Source: three-view drawing plus pictorial views. Frame: mm from the lowest corner of the part. A direction names the side the tool comes from. Round coordinates to 2 decimals unless told otherwise and drop trailing zeros. Loops run counter-clockwise (first coordinate to the right, second up) from the corner with the lowest first, then second, coordinate; pieces in that order, holes last. Notation, with made-up numbers: M 19.25,20.25 L 75.25,20.25 A19 ccw 75.25,56.25 Z; hole C 24.25,-16 d11. An arc over 180 degrees is marked long. Return JSON: item names as keys, results as strings. Group by question number.
1) Contact query for a flat-ended pin moving along its axis: P1, Ø1.5, axis at y = 45.5, z = 15.5, coming from the -X side. Output: stop coordinate, or through.
2) Material intervals for line 1 (X direction, y = 79, z = 18.5); line 2 (Y direction, x = 38.5, z = 9.25); line 3 (Y direction, x = 14.5, z = 3), sorted ascending. Write a range as from..to.
3) Section D-D (z = 2). Output: boundary loops of the cut face in (x, y).
4) Section B-B (z = 8.25). Output: boundary loops of the cut face in (x, y), plus the area to 3 significant figures.
5) Section C-C (y = 16.5). Output: boundary loops of the cut face in (x, z).
6) Access query for the marked faces 1 and 2. Directions: +Z, -Z, +X, -X, +Y, -Y. A direction counts if a zero-diameter tool reaches every point of the face in a straight line with its end or side. Return the directions, or none.
7) Section A-A (y = 140.5). Output: boundary loops of the cut face in (x, z).
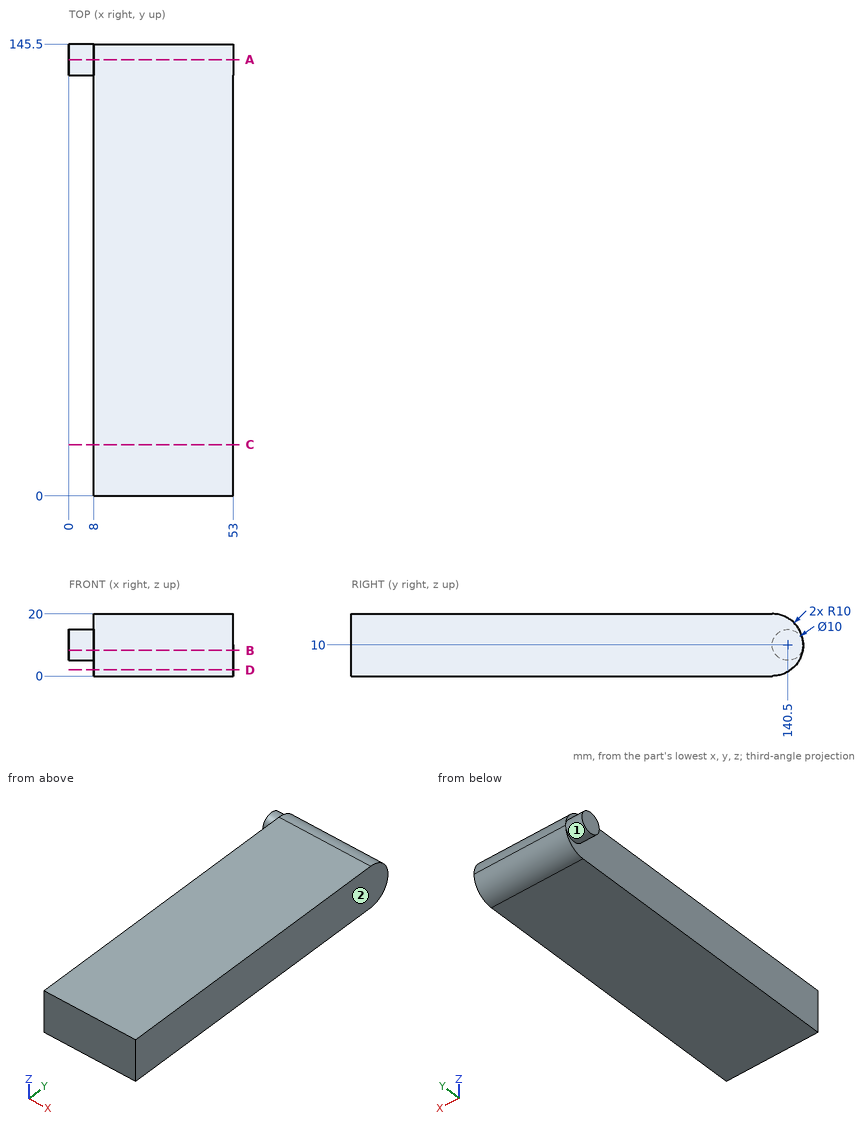
Returned:
{
 "1": {"P1": "stops at x = 8"},
 "2": {"line 1": "x = 8..53", "line 2": "y = 0..145.47", "line 3": "y = 0..142.64"},
 "3": {"outline": "M 8,0 L 53,0 L 53,141.5 L 8,141.5 Z"},
 "4": {"outline": "M 0,135.82 L 8,135.82 L 8,0 L 53,0 L 53,145.35 L 8,145.35 L 8,145.18 L 0,145.18 Z", "area": "6,620 mm^2"},
 "5": {"outline": "M 8,0 L 53,0 L 53,20 L 8,20 Z"},
 "6": {"face 1": "-X", "face 2": "+Z, -Z, +X, +Y, -Y"},
 "7": {"outline": "M 0,5 L 8,5 L 8,1.34 L 53,1.34 L 53,18.66 L 8,18.66 L 8,15 L 0,15 Z"}
}
